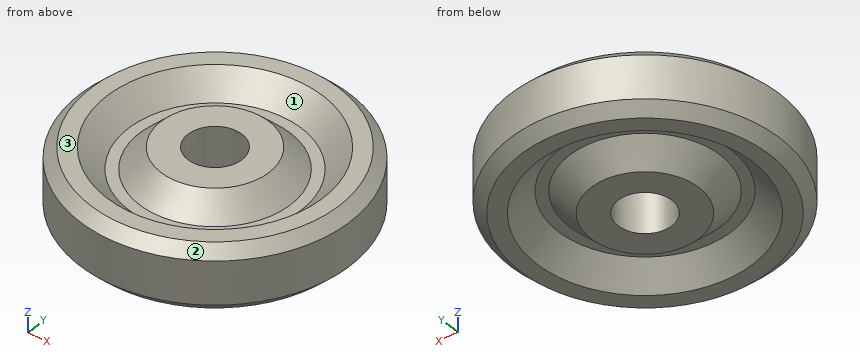
from build123d import *

# Parameters (mm, degrees)
SKETCH2_R                 = 12.5
BOSS_EXTRUDE1_DEPTH       = 3
SKETCH3_R                 = 2.5
CUT_EXTRUDE1_DEPTH        = 6
SKETCH4_R                 = 10
SKETCH4_R_2               = 5
CUT_EXTRUDE2_DEPTH        = 2
CUT_EXTRUDE2_DRAFT        = -45
MIRROR1_COPY_1_SKETCH_R   = 10
MIRROR1_COPY_1_SKETCH_R_2 = 5
MIRROR1_COPY_1_DEPTH      = 2
MIRROR1_COPY_1_DRAFT      = -45
CHAMFER1_SIZE             = 1


with BuildPart() as part:
    # Sketch2 → Boss-Extrude1 (new, symmetric)
    with BuildSketch(Plane.XY):
        Circle(SKETCH2_R)
    extrude(amount=BOSS_EXTRUDE1_DEPTH, both=True)

    # Sketch3 → Cut-Extrude1 (cut)
    with BuildSketch(Plane.XY.offset(3)):
        Circle(SKETCH3_R)
    extrude(amount=-CUT_EXTRUDE1_DEPTH, mode=Mode.SUBTRACT)


with BuildPart() as cut_extrude2_tool:
    # Sketch4 → Cut-Extrude2 (with draft: the straight prism first)
    with BuildSketch(Plane.XY.offset(3)):
        Circle(SKETCH4_R)
        Circle(SKETCH4_R_2, mode=Mode.SUBTRACT)
    extrude(amount=-CUT_EXTRUDE2_DEPTH)
    # Cut-Extrude2: the draft: its side faces are tilted about the plane it starts from
    cut_extrude2_sides = [cut_extrude2_tool.faces().sort_by_distance(p)[0] for p in [
        (-10, 0, 2),
        (-5, 0, 2),
    ]]
    draft(cut_extrude2_sides, Plane.XY.offset(3), CUT_EXTRUDE2_DRAFT)


with BuildPart() as part_1:
    add(part.part)

    # Cut-Extrude2: cut by cut_extrude2_tool
    add(cut_extrude2_tool.part, mode=Mode.SUBTRACT)


with BuildPart() as mirror1_copy_1_tool:
    # Mirror1 copy 1 sketch → Mirror1 copy 1 (with draft: the straight prism first)
    with BuildSketch(Plane(origin=(0, 0, -3), x_dir=(1, 0, 0), z_dir=(0, 0, -1))):
        Circle(MIRROR1_COPY_1_SKETCH_R)
        Circle(MIRROR1_COPY_1_SKETCH_R_2, mode=Mode.SUBTRACT)
    extrude(amount=-MIRROR1_COPY_1_DEPTH)
    # Mirror1 copy 1: the draft: its side faces are tilted about the plane it starts from
    mirror1_copy_1_sides = [mirror1_copy_1_tool.faces().sort_by_distance(p)[0] for p in [
        (-10, 0, -2),
        (-5, 0, -2),
    ]]
    draft(mirror1_copy_1_sides, Plane(origin=(0, 0, -3), x_dir=(1, 0, 0), z_dir=(0, 0, -1)), MIRROR1_COPY_1_DRAFT)


with BuildPart() as part_2:
    add(part_1.part)

    # Mirror1 copy 1: cut by mirror1_copy_1_tool
    add(mirror1_copy_1_tool.part, mode=Mode.SUBTRACT)

    # Chamfer1
    chamfer1_edges = [part_2.edges().sort_by_distance(p)[0] for p in [
        (-12.5, 0, -3),
        (-12.5, 0, 3),
    ]]
    chamfer(chamfer1_edges, length=CHAMFER1_SIZE)


solid = part_2.part
Here's how the part is built. I have some questions about the finished solid (model axes, mm). Face numbers are marked on the shaded views. Give positions to 0.01 mm unless a question says otherwise; leave off trailing zeros. Order: outer loops, then holes, each group sorted by start corner. A loop starts at its lowest first (then second) coordinate and runs counter-clockwise, first axis right, second up. Notation, with made-up numbers: (-12, 6) -> (-7, 6) arc R22 cw to (-7, 43) -> close; hole circle Ø3 at (-13, 80.25). An arc over 180 degrees is marked (long way). One line per item, written item: value. Start each with the question number.
1. Imagine slicing it at A-A, the plane x = 0. List the corners of the cut face in (y, z) for me, plus the area to 3 significant figures.
2. Will these pins go through, and if not, where does the flat tip stop? pin 1 Ø1 at (x, z) = (4.5, 1) entering from +Y; pin 2 Ø1.5 at (y, z) = (-10, -1) entering from +X; pin 3 Ø2 at (x, z) = (2.5, 0.5) entering from +Y; pin 4 Ø8 at (x, y) = (-3.5, 6.5) entering from -Z.
3. I need wall thicknesses on probe 1 along Y at (x, z) = (0, -1.05); probe 2 along X at (y, z) = (-1, 2.35); probe 3 along Y at (x, z) = (0, -0.15). Which ranges of each line are inside material? Lowest first, please. Write a range as from..to.
4. We'd pull the mould along X, two halves only. Please class the marked faces 1, 2 and 3: released by +X, released by -X, zero draft, split by the parting line, or undercut.
5. Imagine slicing it at C-C, the plane z = 0.7. List the corners of the cut face in (x, y) for me.
Values follow:
1. outline: (-12.5, -2) -> (-11.5, -3) -> (-10, -3) -> (-8, -1) -> (-7, -1) -> (-5, -3) -> (-2.5, -3) -> (-2.5, 3) -> (-5, 3) -> (-7, 1) -> (-8, 1) -> (-10, 3) -> (-11.5, 3) -> (-12.5, 2) -> close; (2.5, -3) -> (5, -3) -> (7, -1) -> (8, -1) -> (10, -3) -> (11.5, -3) -> (12.5, -2) -> (12.5, 2) -> (11.5, 3) -> (10, 3) -> (8, 1) -> (7, 1) -> (5, 3) -> (2.5, 3) -> close
1. area: 94.0 mm2
2. pin 1: stops at y = 11.84
2. pin 2: stops at x = 8.41
2. pin 3: stops at y = 12.41
2. pin 4: stops at z = -3
3. probe 1: y = -12.5..-8.05, -6.95..-2.5, 2.5..6.95, 8.05..12.5
3. probe 2: x = -12.11..-9.3, -5.56..-2.29, 2.29..5.56, 9.3..12.11
3. probe 3: y = -12.5..-2.5, 2.5..12.5
4. face 1: undercut
4. face 2: split by the parting line
4. face 3: zero draft
5. outline: circle Ø25 at (0, 0); hole circle Ø5 at (0, 0)
